Here's how the part is built. I have some questions about the finished solid (model axes, mm). Face numbers are marked on the shaded views. Give positions to 0.01 mm unless a question says otherwise; leave off trailing zeros. Order: outer loops, then holes, each group sorted by start corner. A loop starts at its lowest first (then second) coordinate and runs counter-clockwise, first axis right, second up. Notation, with made-up numbers: (-1, -5) -> (39, -5) arc R31 cw to (39, 31) -> close; hole circle Ø6 at (-33.5, 1.5). An arc over 180 degrees is marked (long way). Write each question's results on one line, items separated by ' | '. Start each with the question number.
Q1. Imagine slicing it at D-D, the plane x = 9.5. Please give me the cut outline in (y, z).
Q2. I need wall thicknesses on line 1 along Y through (x, z) = (14.8, -2.2); line 2 along Y through (x, z) = (14.8, -1.6); line 3 along Z through (x, y) = (26, 38). Which ranges of each line are inside material? Lowest first, please. Write a range as [from, to].
Q3. Imagine slicing it at C-C, the plane x = 14.8. Please give me the cut outline in (y, z).
Q4. I'm going to push flat-ended pins straight in: pin 1 (0.8 mm diameter, centred on y = 35.5, z = -2.5, fed in from +X); pin 2 (4.5 mm diameter, centred on x = 14.8, y = 38.8, fed in from +Z); pin 3 (0.5 mm diameter, centred on y = 40.5, z = -2.5, fed in from -X). Where does each tip first touch, or does it pass through?
Q5. Imagine slicing it at A-A, the plane y = 38.8. Please give me the cut outline in (x, z), then the cut area to 3 significant figures.
Q6. Thinking about a two-plate mould opening in X: for the marked faces 1, 2 and 3, which applies, pulls with the +X half, pulls with the -X half, needs draft (parallel to the pull), parting line crosses it, or undercut?
Q7. Imagine slicing it at B-B, the plane z = -0.6. Please give me the cut outline in (x, y).
Autodesk Inventor part; units mm, degrees
ref_plane "YZ Plane" through (0, 0, 0) normal (1, 0, 0) x (0, 1, 0)
ref_plane "XZ Plane" through (0, 0, 0) normal (0, 1, 0) x (-1, 0, 0)
ref_plane "XY Plane" through (0, 0, 0) normal (0, 0, 1) x (1, 0, 0)
sketch "Skizze1" plane through (0, 0, 0) normal (0, 0, 1) x (1, 0, 0)
  line L0 (0, 0) -> (27, 0)
  line L1 (27, 0) -> (27, 59)
  line L2 (27, 59) -> (0, 59)
  line L3 (0, 59) -> (0, 0)
  dimension "d0" = 27
  dimension "d1" = 59
extrude "Extrusion1" add sketch "Skizze1" against normal blind 2
sketch "Skizze2" plane through (0, 0, -2) normal (0, 0, -1) x (-1, 0, 0)
  line L0 (-2, 2) -> (-25, 2)
  line L1 (-25, 2) -> (-25, 57)
  line L2 (-25, 57) -> (-2, 57)
  line L3 (-2, 57) -> (-2, 2)
  line L4 (0, 0) -> (0, 59) construction
  line L5 (-27, 0) -> (0, 0) construction
  point P0 (-2, 29.5)
  point P1 (0, 29.5)
  point P2 (-13.5, 2)
  point P3 (-13.5, 0)
  dimension "d4" = 2
  dimension "d5" = 2
extrude "Extrusion2" add sketch "Skizze2" along normal blind 2
sketch "Skizze3" plane through (0, 0, -4) normal (0, 0, -1) x (-1, 0, 0)
  circle A0 centre (-14.8, 38.8) radius 2.5
  line L0 (-27, 0) -> (0, 0)
  line L1 (-2, 2) -> (-2, 57)
  line L2 (-25, 57) -> (-25, 2)
  circle A1 centre (-14.8, 46.42) radius 2.5
  dimension "d8" = 5
  dimension "d9" = 38.8
  dimension "d11" = 10.2
  dimension "d12" = 5
  dimension "d13" = 7.62
extrude "Extrusion3" cut sketch "Skizze3" against normal through all
fillet "Rundung1" radius 1 4 edges at (13.5, 57, -4) (25, 29.5, -4) (2, 29.5, -4) (13.5, 2, -4)
fillet "Rundung2" radius 2 4 edges at (0, 59, -1) (0, 0, -1) (27, 59, -1) (27, 0, -1)
properties part number "top"
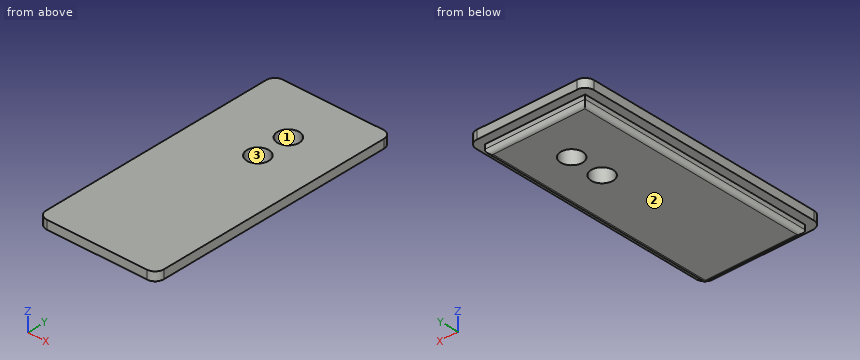
Geometry check:
1) outline: (0, -2) -> (2, -2) -> (2, -3) arc R1 ccw to (3, -4) -> (56, -4) arc R1 ccw to (57, -3) -> (57, -2) -> (59, -2) -> (59, 0) -> (0, 0) -> close
2) line 1: [2, 36.3], [41.3, 43.92], [48.92, 57] | line 2: [0, 36.3], [41.3, 43.92], [48.92, 59] | line 3: [-2, 0]
3) outline: (0, -2) -> (2, -2) -> (2, -3) arc R1 ccw to (3, -4) -> (36.3, -4) -> (36.3, 0) -> (0, 0) -> close; (41.3, -4) -> (43.92, -4) -> (43.92, 0) -> (41.3, 0) -> close; (48.92, -4) -> (56, -4) arc R1 ccw to (57, -3) -> (57, -2) -> (59, -2) -> (59, 0) -> (48.92, 0) -> close
4) pin 1: x = 25 | pin 2: through | pin 3: x = 2
5) outline: (0, -2) -> (2, -2) -> (2, -3) arc R1 ccw to (3, -4) -> (12.3, -4) -> (12.3, 0) -> (0, 0) -> close; (17.3, -4) -> (24, -4) arc R1 ccw to (25, -3) -> (25, -2) -> (27, -2) -> (27, 0) -> (17.3, 0) -> close | area: 79.6 mm²
6) face 1: undercut | face 2: needs draft | face 3: undercut
7) outline: (0, 2) arc R2 ccw to (2, 0) -> (25, 0) arc R2 ccw to (27, 2) -> (27, 57) arc R2 ccw to (25, 59) -> (2, 59) arc R2 ccw to (0, 57) -> close; hole circle Ø5 at (14.8, 38.8); hole circle Ø5 at (14.8, 46.42)
